The model under review builds one solid part; all positions refer to its coordinate system, in mm. Face numbers are marked on the shaded views. A direction names the side the tool comes from. Coordinates: 2 decimals unless noted, no trailing zeros. Write each loop counter-clockwise with the first axis right and the second up, starting at its lowest first coordinate (ties: lowest second). Pieces come first, ordered by that corner, then holes. Notation, with made-up numbers: (-12.5, 80.25) - (19.5, 80.25) arc R12 ccw to (19.5, 96.25) - close; hole circle Ø1 at (70, 37.25). An arc over 180 degrees is marked (long way). Put each result on its own line as item: value.
from build123d import *

# Parameters (mm, degrees)
SKETCH_W     = 12.2
SKETCH_H     = 9
PAD_DEPTH    = 1.6
SKETCH001_W  = 8.7
SKETCH001_H  = 3.8
PAD001_DEPTH = 3.9
SKETCH002_W  = 1.5
SKETCH002_H  = 1.5
PAD002_DEPTH = 1.4


with BuildPart() as part:
    # Sketch → Pad (new body)
    with BuildSketch(Plane.XY):
        Rectangle(SKETCH_W, SKETCH_H)
    extrude(amount=PAD_DEPTH)

    # Sketch001 → Pad001 (new body)
    with BuildSketch(Plane.XY.offset(1.6)):
        Rectangle(SKETCH001_W, SKETCH001_H)
    extrude(amount=PAD001_DEPTH)

    # Sketch002 → Pad002 (new body)
    with BuildSketch(Plane.XY.offset(5.5)):
        with Locations((2.15, 0)):
            Rectangle(SKETCH002_W, SKETCH002_H)
    extrude(amount=PAD002_DEPTH)


solid = part.part
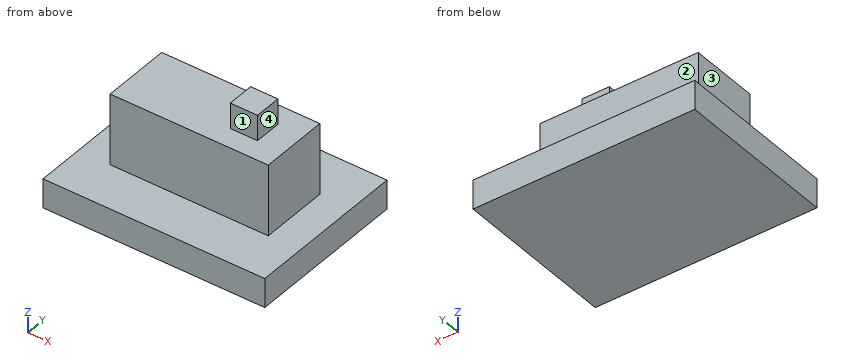
1. Consider section C-C on y = -0.25. State the section outline as (x, z) points.
Determined:
outline: (-6.1, 0) - (6.1, 0) - (6.1, 1.6) - (4.35, 1.6) - (4.35, 5.5) - (2.9, 5.5) - (2.9, 6.9) - (1.4, 6.9) - (1.4, 5.5) - (-4.35, 5.5) - (-4.35, 1.6) - (-6.1, 1.6) - close
2. To check wall thickness, follow probe 1 along Y at (x, z) = (2.5, 2); probe 2 along Z at (x, y) = (2, 1.5); probe 3 along X at (y, z) = (0.25, 6.25). State the ranges of each line that lie inside material, in increasing order.
Determined:
probe 1: y = -1.9 to 1.9
probe 2: z = 0 to 5.5
probe 3: x = 1.4 to 2.9
3. Machinability: for the marked faces 1, 2, 3 and 4, which of the approach directions +Z, -Z, +X, -X, +Y, -Y give a long, thin tool a straight path to every point of the face, cutting with its end or side? Answer none if there is none.
Determined:
face 1: +Z, +X, -X, -Y
face 2: +Z, +X, -X, +Y
face 3: +Z, -X, +Y, -Y
face 4: +Z, +X, +Y, -Y
4. Consider section A-A on y = 1.75. State the section outline as (x, z) points.
Determined:
outline: (-6.1, 0) - (6.1, 0) - (6.1, 1.6) - (4.35, 1.6) - (4.35, 5.5) - (-4.35, 5.5) - (-4.35, 1.6) - (-6.1, 1.6) - close
5. Consider section D-D on z = 2.25. State the section outline as (x, y) points, plus the area to 3 significant figures.
Determined:
outline: (-4.35, -1.9) - (4.35, -1.9) - (4.35, 1.9) - (-4.35, 1.9) - close
area: 33.1 mm^2
6. Consider section B-B on x = 2.5. State the section outline as (y, z) points, plus the area to 3 significant figures.
Determined:
outline: (-4.5, 0) - (4.5, 0) - (4.5, 1.6) - (1.9, 1.6) - (1.9, 5.5) - (0.75, 5.5) - (0.75, 6.9) - (-0.75, 6.9) - (-0.75, 5.5) - (-1.9, 5.5) - (-1.9, 1.6) - (-4.5, 1.6) - close
area: 31.3 mm^2
7. For pin 1 Ø1.5 at (y, z) = (0, 6) entering from +X; pin 2 Ø2 at (x, z) = (-1, 3) entering from +Y; pin 3 Ø1.5 at (y, z) = (-0.5, 6) entering from -X, all flat-tipped, find the tip position at first contact; note any pin that passes through.
Determined:
pin 1: stops at x = 4.35
pin 2: stops at y = 1.9
pin 3: stops at x = -4.35
